Design review of the part shown in the three views and the two pictorial views. Dimensions are in mm from the part's minimum x, y and z. A direction names the side the tool comes from. Give positions to 0.01 mm unless a question says otherwise; leave off trailing zeros. Loops run counter-clockwise (first coordinate to the right, second up) from the corner with the lowest first, then second, coordinate; pieces in that order, holes last.
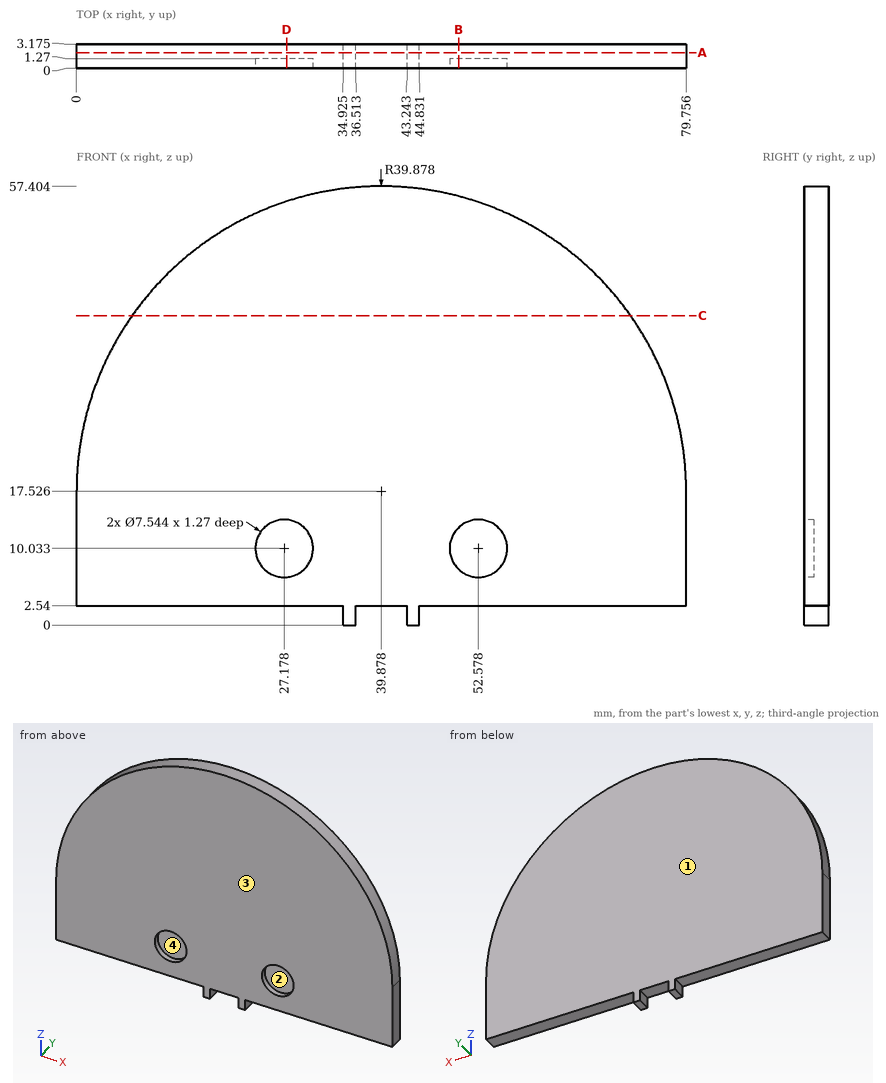
Q1. Wall thickness on line 1 (X direction, y = 2.5, z = 18); line 2 (Z direction, x = 28, y = 0.5) (1 decimal); line 3 (Z direction, x = 17, y = 2.35): over which ranges is each line inside the solid? List them lowest first.
Results:
line 1: x = 0 to 79.75
line 2: z = 2.5 to 6.4, 13.7 to 55.6
line 3: z = 2.54 to 50.19
Q2. Tool access review of the marked faces 3 and 4: name each direction out of +Z, -Z, +X, -X, +Y, -Y from which nothing blocks a thin tool from reaching the whole face with its end or side.
Results:
face 3: +Z, -Z, +X, -X, -Y
face 4: -Y
Q3. Insertion check: pin 1 (1.5 mm diameter, centred on y = 2.5, z = 51.5, fed in from -X) (1 decimal); pin 2 (4.5 mm diameter, centred on x = 52.578, z = 10.033, fed in from -Y); pin 3 (2 mm diameter, centred on x = 67.5, z = 7, fed in from -Y); pin 4 (1.3 mm diameter, centred on y = 2, z = 1, fed in from -X) (1 decimal). Each pin has a flat end and moves straight along its axis. Give the tip position at first contact, or say it passes through.
Results:
pin 1: stops at x = 17.8
pin 2: stops at y = 1.27
pin 3: stops at y = 0
pin 4: stops at x = 34.9
Q4. Take a section at B-B (x = 50). Give the boundary of the cut face in (y, z) (1 decimal).
Results:
outline: (0, 2.5) - (3.2, 2.5) - (3.2, 56.1) - (0, 56.1) - (0, 12.8) - (1.3, 12.8) - (1.3, 7.3) - (0, 7.3) - close
Q5. Take a section at D-D (x = 27.5). Give the boundary of the cut face in (y, z) (1 decimal).
Results:
outline: (0, 2.5) - (3.2, 2.5) - (3.2, 55.4) - (0, 55.4) - (0, 13.8) - (1.3, 13.8) - (1.3, 6.3) - (0, 6.3) - close
Q6. Take a section at C-C (z = 40.5). Give the boundary of the cut face in (x, y) (1 decimal).
Results:
outline: (7.3, 0) - (72.5, 0) - (72.5, 3.2) - (7.3, 3.2) - close
Q7. Take a section at A-A (y = 2.05). Give the boundary of the cut face in (x, z) (1 decimal), plus the area to 3 significant figures.
Results:
outline: (0, 2.5) - (34.9, 2.5) - (34.9, 0) - (36.5, 0) - (36.5, 2.5) - (43.2, 2.5) - (43.2, 0) - (44.8, 0) - (44.8, 2.5) - (79.8, 2.5) - (79.8, 17.5) arc R39.9 ccw to (0, 17.5) - close
area: 3,700 mm2
Q8. Draft analysis for pull direction Z (two halves, no side actions). For the marked faces 1 and 2, state which applies: pulls with the +Z half, pulls with the -Z half, needs draft (parallel to the pull), parting line crosses it, or undercut.
Results:
face 1: needs draft
face 2: undercut
